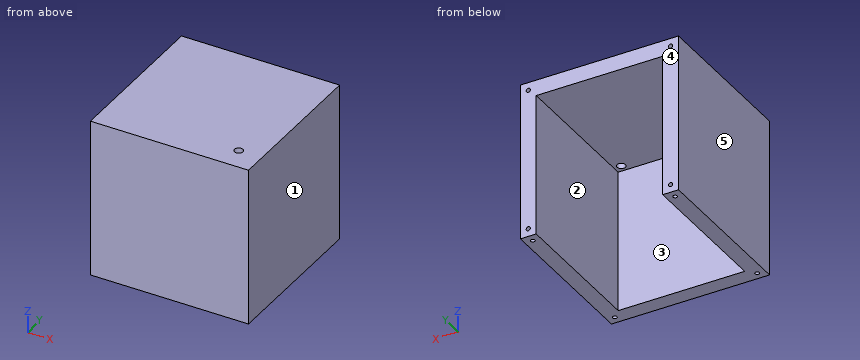
```python
from build123d import *

# Parameters (mm, degrees)
CROQUIS1_W              = 150
CROQUIS1_H              = 150
SALIENTE_EXTRUIR1_DEPTH = 150
CROQUIS2_W              = 120
CROQUIS2_H              = 15
CROQUIS2_H_2            = 120
CORTAR_EXTRUIR1_DEPTH   = 135
CROQUIS3_R              = 2
CORTAR_EXTRUIR2_DEPTH   = 10
CROQUIS4_R              = 2
CORTAR_EXTRUIR3_DEPTH   = 10
CROQUIS5_R              = 4
CORTAR_EXTRUIR4_DEPTH   = 15


with BuildPart() as part:
    # Croquis1 → Saliente-Extruir1 (new body)
    with BuildSketch(Plane.XY):
        Rectangle(CROQUIS1_W, CROQUIS1_H)
    extrude(amount=SALIENTE_EXTRUIR1_DEPTH)

    # Croquis2 → Cortar-Extruir1 (cut)
    with BuildSketch(Plane(origin=(0, 0, 0), x_dir=(-1, 0, 0), z_dir=(0, 0, -1))):
        with Locations((0, 67.5)):
            Rectangle(CROQUIS2_W, CROQUIS2_H)
        Rectangle(CROQUIS2_W, CROQUIS2_H_2)
    extrude(amount=-CORTAR_EXTRUIR1_DEPTH, mode=Mode.SUBTRACT)

    # Croquis3 → Cortar-Extruir2 (cut)
    with BuildSketch(Plane(origin=(0, 75, 0), x_dir=(1, 0, 0), z_dir=(0, 1, 0))):
        with Locations(Location((-67.5, -142.5, 0), (0, 0, 270))):
            Circle(CROQUIS3_R)
        with Locations(Location((67.5, -142.5, 0), (0, 0, 270))):
            Circle(CROQUIS3_R)
        with Locations(Location((67.5, -7.5, 0), (0, 0, 270))):
            Circle(CROQUIS3_R)
        with Locations(Location((-67.5, -7.5, 0), (0, 0, 270))):
            Circle(CROQUIS3_R)
    extrude(amount=-CORTAR_EXTRUIR2_DEPTH, mode=Mode.SUBTRACT)

    # Croquis4 → Cortar-Extruir3 (cut)
    with BuildSketch(Plane(origin=(0, 0, 0), x_dir=(-1, 0, 0), z_dir=(0, 0, -1))):
        with Locations((-67.5, -67.5)):
            Circle(CROQUIS4_R)
        with Locations((67.5, -67.5)):
            Circle(CROQUIS4_R)
        with Locations((67.5, 67.5)):
            Circle(CROQUIS4_R)
        with Locations((-67.5, 67.5)):
            Circle(CROQUIS4_R)
    extrude(amount=-CORTAR_EXTRUIR3_DEPTH, mode=Mode.SUBTRACT)

    # Croquis5 → Cortar-Extruir4 (cut)
    with BuildSketch(Plane.XY.offset(150)):
        with Locations((53.033008589, -53.033008589)):
            Circle(CROQUIS5_R)
    extrude(amount=-CORTAR_EXTRUIR4_DEPTH, mode=Mode.SUBTRACT)


solid = part.part
```
The listing builds one solid part. Answer for the finished solid, in the listing's coordinates (mm). Face numbers are marked on the shaded views. A direction names the side the tool comes from. Give positions to 0.01 mm unless a question says otherwise; leave off trailing zeros. Order: outer loops, then holes, each group sorted by start corner. A loop starts at its lowest first (then second) coordinate and runs counter-clockwise, first axis right, second up.
Item 1: Find the intervals of material crossed by probe 1 along X at (y, z) = (70.75, 7.5); probe 2 along Y at (x, z) = (-67.5, 2.25); probe 3 along X at (y, z) = (66, 127), in increasing order.
From the geometry:
probe 1: x = -75 to -69.5, -65.5 to -60, 60 to 65.5, 69.5 to 75
probe 2: y = -75 to -69.5, -65.5 to 65.5, 69.5 to 75
probe 3: x = -75 to -60, 60 to 75
Item 2: The part is cut by section C-C, the plane x = 18.5. Give the vertices of the cut face in (y, z).
From the geometry:
outline: (-75, 0) - (-60, 0) - (-60, 135) - (75, 135) - (75, 150) - (-75, 150) - close
Item 3: Given pin 1 Ø1.2 at (x, z) = (-67.5, 143) entering from +Y; pin 2 Ø4 at (x, y) = (6, -44.5) entering from -Z; pin 3 Ø2.5 at (x, y) = (-67.5, -67.5) entering from -Z, each flat-ended and moving along its own axis, determine where each tip first touches the part or whether it passes through.
From the geometry:
pin 1: stops at y = 65
pin 2: stops at z = 135
pin 3: stops at z = 10
Item 4: For a pull along X with two mould halves and no side action, classify the marked faces 3, 4 and 5 as pulls with the +X half, pulls with the -X half, needs draft (parallel to the pull), parting line crosses it, or undercut.
From the geometry:
face 3: undercut
face 4: needs draft
face 5: pulls with the -X half
Item 5: The part is cut by section A-A, the plane y = -41.5. Give the vertices of the cut face in (x, z).
From the geometry:
outline: (-75, 0) - (-60, 0) - (-60, 135) - (60, 135) - (60, 0) - (75, 0) - (75, 150) - (-75, 150) - close
Item 6: The part is cut by section B-B, the plane z = 126.5. Give the vertices of the cut face in (x, y).
From the geometry:
outline: (-75, -75) - (75, -75) - (75, 75) - (60, 75) - (60, -60) - (-60, -60) - (-60, 75) - (-75, 75) - close
Item 7: Which of the six approach directions +Z, -Z, +X, -X, +Y, -Y give full straight-line access (tool end or side, diameter ignored) to the marked faces 1 and 2?
From the geometry:
face 1: +Z, -Z, +X, +Y, -Y
face 2: -Z, +Y
